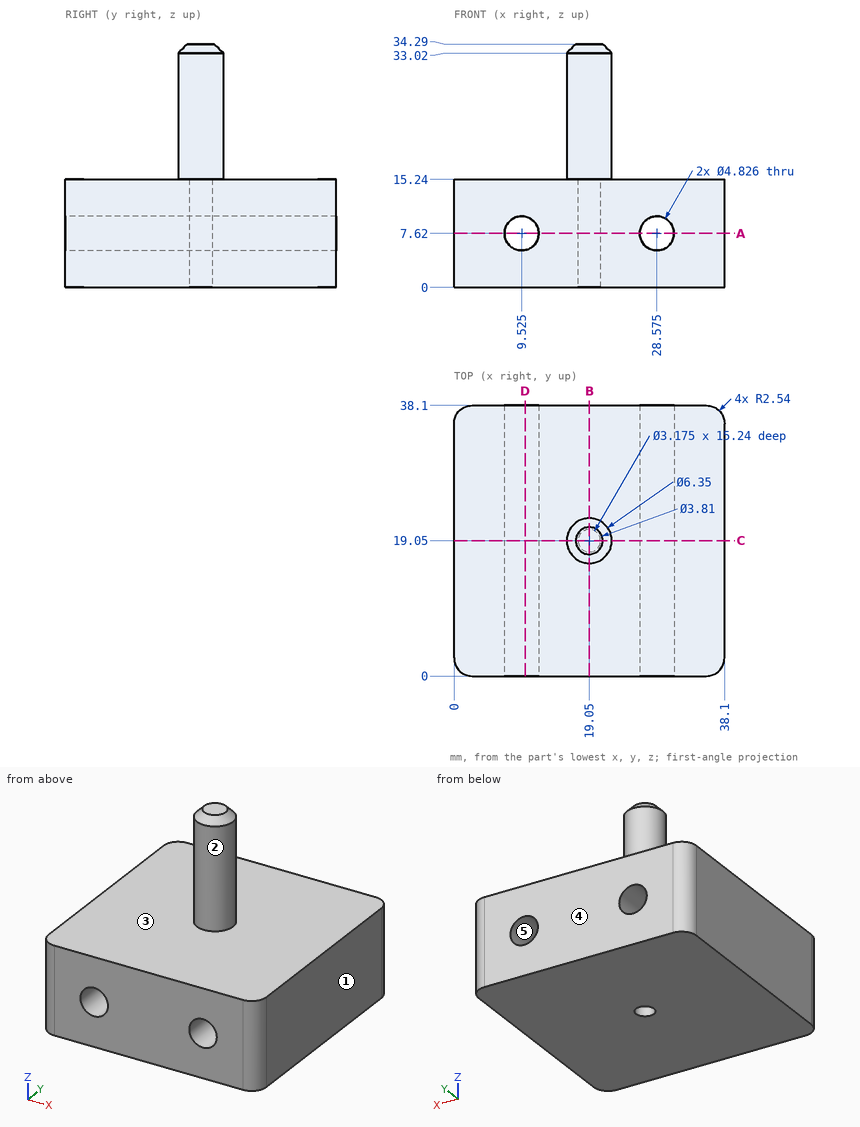
Study the drawing (mm; zero at the part's minimum x, y, z) and answer. A direction names the side the tool comes from. Coordinates: 2 decimals unless noted, no trailing zeros. Write each loop counter-clockwise with the first axis right and the second up, starting at its lowest first coordinate (ties: lowest second). Pieces come first, ordered by that corner, then holes.
Q1. Given P1, Ø5, axis at x = 18.5, y = 33.5, coming from the +Z side; P2, Ø8, axis at x = 17, z = 19.5, coming from the +Y side (3 decimals), each flat-ended and moving along its own axis, determine where each tip first touches the part or whether it passes through.
Returned:
P1: stops at z = 15.24
P2: stops at y = 22.225
Q2. Find the intervals of material crossed by line 1 along X through (y, z) = (29, 7.5); line 2 along Y through (x, z) = (19.05, 12); line 3 along Z through (x, y) = (23, 27), in increasing order.
Returned:
line 1: x = 0 to 7.11, 11.94 to 26.16, 30.99 to 38.1
line 2: y = 0 to 17.46, 20.64 to 38.1
line 3: z = 0 to 15.24
Q3. Section C-C, the plane y = 19.05 is taken. Write down the section's boundary in (x, z) (1 decimal).
Returned:
outline: (0, 0) - (17.5, 0) - (17.5, 15.2) - (20.6, 15.2) - (20.6, 0) - (38.1, 0) - (38.1, 15.2) - (22.2, 15.2) - (22.2, 33) - (21, 34.3) - (17.1, 34.3) - (15.9, 33) - (15.9, 15.2) - (0, 15.2) - close; hole circle Ø4.8 at (9.5, 7.6); hole circle Ø4.8 at (28.6, 7.6)
Q4. The mould has two halves that part along Z. Classify the marked faces 3, 4 and 5: released by +Z, released by -Z, zero draft, split by the parting line, or undercut.
Returned:
face 3: released by +Z
face 4: zero draft
face 5: undercut
Q5. Section D-D, the plane x = 10 is taken. Write down the section's boundary in (y, z), then the cut area to 3 significant figures.
Returned:
outline: (0, 0) - (38.1, 0) - (38.1, 5.25) - (0, 5.25) - close; (0, 9.99) - (38.1, 9.99) - (38.1, 15.24) - (0, 15.24) - close
area: 400 mm2
Q6. Which of the six approach directions +Z, -Z, +X, -X, +Y, -Y give full straight-line access (tool end or side, diameter ignored) to the marked faces 1 and 2?
Returned:
face 1: +Z, -Z, +X, +Y, -Y
face 2: +Z
Q7. Section A-A, the plane z = 7.62 is taken. Give the number of separate pieces and of enclosed holes in the cut face, then the cut area to 3 significant figures.
Returned:
separate pieces: 3
enclosed holes: 1
area: 1,070 mm2
Q8. Section B-B, the plane x = 19.05 is taken. Write down the section's boundary in (y, z) (1 decimal).
Returned:
outline: (0, 0) - (17.5, 0) - (17.5, 15.2) - (20.6, 15.2) - (20.6, 0) - (38.1, 0) - (38.1, 15.2) - (22.2, 15.2) - (22.2, 33) - (21, 34.3) - (17.1, 34.3) - (15.9, 33) - (15.9, 15.2) - (0, 15.2) - close
